Read the model definition and answer for the solid it produces. Units are mm, in the model's axes. A direction names the side the tool comes from. Round coordinates to 2 decimals unless told otherwise and drop trailing zeros.
from build123d import *

# Parameters (mm, degrees)
SKETCH2_W            = 37
SKETCH2_H            = 37
BOSS_EXTRUDE1_DEPTH  = 3
SKETCH3_R            = 6
BOSS_EXTRUDE2_DEPTH  = 2.3
SKETCH6_R            = 18.5
SKETCH6_R_2          = 8.5
BOSS_EXTRUDE3_DEPTH  = 2.3
CUT_EXTRUDE2_DEPTH   = 2.3
CIRPATTERN1_COUNT    = 4
CUT_EXTRUDE3_DEPTH   = 2.3
CIRPATTERN2_COUNT    = 4
CUT_EXTRUDE5_DEPTH   = 3
CIRPATTERN7_COUNT    = 4
MIRROR2_COPY_1_DEPTH = 3
MIRROR2_COPY_2_DEPTH = 3
MIRROR2_COPY_3_DEPTH = 3
SKETCH11_R           = 6.25
BOSS_EXTRUDE4_DEPTH  = 3
CIRPATTERN9_COUNT    = 2
CIRPATTERN9_ANGLE    = 90
SKETCH12_R           = 5
BOSS_EXTRUDE5_DEPTH  = 2.3
CIRPATTERN10_COUNT   = 2
CIRPATTERN10_ANGLE   = 90
CIRPATTERN11_COUNT   = 2
CIRPATTERN11_ANGLE   = 90
SCALE1_SCALE         = 0.965
SKETCH19_W           = 7
SKETCH19_H           = 6.5
CUT_EXTRUDE6_DEPTH   = 3
SKETCH20_W           = 5.6
SKETCH20_H           = 1.8
CUT_EXTRUDE7_DEPTH   = 1.5
SKETCH28_W           = 7
SKETCH28_H           = 6.5
CUT_EXTRUDE10_DEPTH  = 3
SKETCH30_W           = 5.6
SKETCH30_H           = 1.8
CUT_EXTRUDE11_DEPTH  = 1.5
CIRPATTERN12_COUNT   = 4
SKETCH33_W           = 7
SKETCH33_H           = 6.5
CUT_EXTRUDE12_DEPTH  = 3
SKETCH35_W           = 5.6
SKETCH35_H           = 1.8
CUT_EXTRUDE13_DEPTH  = 1.5
SKETCH37_W           = 7
SKETCH37_H           = 6.5
CUT_EXTRUDE14_DEPTH  = 3
SKETCH39_W           = 5.6
SKETCH39_H           = 1.8
CUT_EXTRUDE15_DEPTH  = 1.5


with BuildPart() as part:
    # Sketch2 → Boss-Extrude1 (new body)
    with BuildSketch(Plane.XY):
        Rectangle(SKETCH2_W, SKETCH2_H)
    extrude(amount=BOSS_EXTRUDE1_DEPTH)

    # Sketch3 → Boss-Extrude2 (add)
    with BuildSketch(Plane.XY.offset(3)):
        Circle(SKETCH3_R)
    extrude(amount=BOSS_EXTRUDE2_DEPTH)

    # Sketch5 → Revolve1 (revolve)
    with BuildSketch(Plane(origin=(0, 0, 0), x_dir=(-1, 0, 0), z_dir=(0, -1, 0))):
        with BuildLine():
            Line((6, -5.3), (0, -5.3))
            Line((0, -5.3), (0, -6.3))
            ThreePointArc((0, -6.3), (3.041381265, -6.048287591), (6, -5.3))
        make_face()
    revolve(axis=Axis((0, 0, 5.3), (0, 0, 1)))

    # Sketch6 → Boss-Extrude3 (add)
    with BuildSketch(Plane.XY.offset(3)):
        Circle(SKETCH6_R)
        Circle(SKETCH6_R_2, mode=Mode.SUBTRACT)
    extrude(amount=BOSS_EXTRUDE3_DEPTH)

    # Sketch8 → Cut-Extrude2 (cut)
    with BuildSketch(Plane.XY.offset(5.3)):
        with BuildLine():
            ThreePointArc((4.25, 7.361215932), (6.01040764, 6.01040764), (7.361215932, 4.25))
            Line((7.361215932, 4.25), (16.02146997, 9.25))
            ThreePointArc((16.02146997, 9.25), (13.081475452, 13.081475452), (9.25, 16.02146997))
            Line((9.25, 16.02146997), (4.25, 7.361215932))
        make_face()
    cut_extrude2 = extrude(amount=-CUT_EXTRUDE2_DEPTH, mode=Mode.SUBTRACT)

    # CirPattern1: Cut-Extrude2 ×4 about axis
    cirpattern1_axis = Axis((0, 0, 5.3), (0, 0, 1))
    for i in range(1, CIRPATTERN1_COUNT):
        add(cut_extrude2.rotate(cirpattern1_axis, i * 360 / CIRPATTERN1_COUNT), mode=Mode.SUBTRACT)

    # Sketch9 → Cut-Extrude3 (cut)
    with BuildSketch(Plane.XY.offset(5.3)):
        with BuildLine():
            Line((16.02146997, 9.25), (12.557368355, 7.25))
            Line((12.557368355, 7.25), (18.043966792, 4.082310915))
            ThreePointArc((18.043966792, 4.082310915), (17.227586832, 6.742421815), (16.02146997, 9.25))
        make_face()
        with BuildLine():
            Line((18.043966792, -4.082310915), (12.557368355, -7.25))
            Line((12.557368355, -7.25), (16.02146997, -9.25))
            ThreePointArc((16.02146997, -9.25), (17.227586832, -6.742421815), (18.043966792, -4.082310915))
        make_face()
    cut_extrude3 = extrude(amount=-CUT_EXTRUDE3_DEPTH, mode=Mode.SUBTRACT)

    # CirPattern2: Cut-Extrude3 ×4 about axis
    cirpattern2_axis = Axis((0, 0, 0), (0, 0, 1))
    for i in range(1, CIRPATTERN2_COUNT):
        add(cut_extrude3.rotate(cirpattern2_axis, i * 360 / CIRPATTERN2_COUNT), mode=Mode.SUBTRACT)

    # Sketch10 → Cut-Extrude5 (cut)
    with BuildSketch(Plane.XY.offset(3)):
        with BuildLine():
            Line((7.447468172, -12.671376657), (4.082310915, -18.5))
            Line((4.082310915, -18.5), (18.5, -18.5))
            Line((18.5, -18.5), (13.378483438, -13.378483438))
            ThreePointArc((13.378483438, -13.378483438), (12.288693225, -13.595256189), (11.671376657, -12.671376657))
            Line((11.671376657, -12.671376657), (7.447468172, -12.671376657))
        make_face()
    cut_extrude5 = extrude(amount=-CUT_EXTRUDE5_DEPTH, mode=Mode.SUBTRACT)

    # CirPattern7: Cut-Extrude5 ×4 about axis
    cirpattern7_axis = Axis((0, 0, 0), (0, 0, 1))
    for i in range(1, CIRPATTERN7_COUNT):
        add(cut_extrude5.rotate(cirpattern7_axis, i * 360 / CIRPATTERN7_COUNT), mode=Mode.SUBTRACT)

    # Mirror2: Cut-Extrude5 across plane
    add(cut_extrude5.mirror(Plane(origin=(0, 0, 0), x_dir=(0, 0, 1), z_dir=(0.707106781, -0.707106781, 0))), mode=Mode.SUBTRACT)

    # Mirror2 copy 1 sketch → Mirror2 copy 1 (cut)
    with BuildSketch(Plane.XY.offset(3)):
        with BuildLine():
            Line((7.447468172, 12.671376657), (4.082310915, 18.5))
            Line((4.082310915, 18.5), (18.5, 18.5))
            Line((18.5, 18.5), (13.378483438, 13.378483438))
            ThreePointArc((13.378483438, 13.378483438), (12.288693225, 13.595256189), (11.671376657, 12.671376657))
            Line((11.671376657, 12.671376657), (7.447468172, 12.671376657))
        make_face()
    extrude(amount=-MIRROR2_COPY_1_DEPTH, mode=Mode.SUBTRACT)

    # Mirror2 copy 2 sketch → Mirror2 copy 2 (cut)
    with BuildSketch(Plane(origin=(0, 0, 3), x_dir=(0, -1, 0), z_dir=(0, 0, 1))):
        with BuildLine():
            Line((7.447468172, 12.671376657), (4.082310915, 18.5))
            Line((4.082310915, 18.5), (18.5, 18.5))
            Line((18.5, 18.5), (13.378483438, 13.378483438))
            ThreePointArc((13.378483438, 13.378483438), (12.288693225, 13.595256189), (11.671376657, 12.671376657))
            Line((11.671376657, 12.671376657), (7.447468172, 12.671376657))
        make_face()
    extrude(amount=-MIRROR2_COPY_2_DEPTH, mode=Mode.SUBTRACT)

    # Mirror2 copy 3 sketch → Mirror2 copy 3 (cut)
    with BuildSketch(Plane(origin=(0, 0, 3), x_dir=(-1, 0, 0), z_dir=(0, 0, 1))):
        with BuildLine():
            Line((7.447468172, 12.671376657), (4.082310915, 18.5))
            Line((4.082310915, 18.5), (18.5, 18.5))
            Line((18.5, 18.5), (13.378483438, 13.378483438))
            ThreePointArc((13.378483438, 13.378483438), (12.288693225, 13.595256189), (11.671376657, 12.671376657))
            Line((11.671376657, 12.671376657), (7.447468172, 12.671376657))
        make_face()
    extrude(amount=-MIRROR2_COPY_3_DEPTH, mode=Mode.SUBTRACT)

    # Sketch11 → Boss-Extrude4 (add)
    with BuildSketch(Plane.XY):
        with Locations((14.849242405, 14.849242405)):
            Circle(SKETCH11_R)
    boss_extrude4 = extrude(amount=BOSS_EXTRUDE4_DEPTH)

    # CirPattern9: Boss-Extrude4 ×2 about axis
    cirpattern9_axis = Axis((0, 0, 5.3), (0, 0, 1))
    for i in range(1, CIRPATTERN9_COUNT):
        add(boss_extrude4.rotate(cirpattern9_axis, i * CIRPATTERN9_ANGLE / (CIRPATTERN9_COUNT - 1)))

    # Sketch12 → Boss-Extrude5 (add)
    with BuildSketch(Plane.XY.offset(3)):
        with Locations((14.849242405, 14.849242405)):
            Circle(SKETCH12_R)
    boss_extrude5 = extrude(amount=BOSS_EXTRUDE5_DEPTH)

    # Sketch14 → Revolve2 (revolve)
    with BuildSketch(Plane(origin=(14.849242405, 0, 0), x_dir=(0, 0, -1), z_dir=(1, 0, 0))):
        with BuildLine():
            Line((-6.3, 14.849242405), (-5.3, 14.849242405))
            Line((-5.3, 14.849242405), (-5.3, 9.849242405))
            ThreePointArc((-5.3, 9.849242405), (-6.047548784, 12.299732648), (-6.3, 14.849242405))
        make_face()
    revolve2 = revolve(axis=Axis((14.849242405, 14.849242405, 5.3), (0, 0, 1)))

    # CirPattern10: Boss-Extrude5 ×2 about axis
    cirpattern10_axis = Axis((0, 0, 5.3), (0, 0, 1))
    for i in range(1, CIRPATTERN10_COUNT):
        add(boss_extrude5.rotate(cirpattern10_axis, i * CIRPATTERN10_ANGLE / (CIRPATTERN10_COUNT - 1)))

    # CirPattern11: Revolve2 ×2 about axis
    cirpattern11_axis = Axis((0, 0, 5.3), (0, 0, 1))
    for i in range(1, CIRPATTERN11_COUNT):
        add(revolve2.rotate(cirpattern11_axis, i * CIRPATTERN11_ANGLE / (CIRPATTERN11_COUNT - 1)))


with BuildPart() as part_1:
    # Scale1: scaled about (0, 0, 0)
    add(part.part.scale(SCALE1_SCALE))

    # Sketch19 → Cut-Extrude6 (cut)
    with BuildSketch(Plane(origin=(0, 0, 0), x_dir=(-1, 0, 0), z_dir=(0, 0, -1))):
        Rectangle(SKETCH19_W, SKETCH19_H)
    extrude(amount=-CUT_EXTRUDE6_DEPTH, mode=Mode.SUBTRACT)

    # Sketch20 → Cut-Extrude7 (cut)
    with BuildSketch(Plane(origin=(0, 0, 0), x_dir=(-1, 0, 0), z_dir=(0, 0, -1))):
        with Locations((0, 4.15)):
            Rectangle(SKETCH20_W, SKETCH20_H)
        with Locations((0, -4.15)):
            Rectangle(SKETCH20_W, SKETCH20_H)
    extrude(amount=-CUT_EXTRUDE7_DEPTH, mode=Mode.SUBTRACT)

    # Sketch28 → Cut-Extrude10 (cut)
    with BuildSketch(Plane(origin=(-9.998493026, 1.351076982, 0), x_dir=(-1, 0, 0), z_dir=(0, 0, -1))):
        with Locations((1.751506974, -1.351076982)):
            Rectangle(SKETCH28_W, SKETCH28_H)
    cut_extrude10 = extrude(amount=-CUT_EXTRUDE10_DEPTH, mode=Mode.SUBTRACT)

    # Sketch30 → Cut-Extrude11 (cut)
    with BuildSketch(Plane(origin=(-9.998493026, 1.351076982, 0), x_dir=(-1, 0, 0), z_dir=(0, 0, -1))):
        with Locations((1.751506974, 2.798923018)):
            Rectangle(SKETCH30_W, SKETCH30_H)
        with Locations((1.751506974, -5.501076982)):
            Rectangle(SKETCH30_W, SKETCH30_H)
    cut_extrude11 = extrude(amount=-CUT_EXTRUDE11_DEPTH, mode=Mode.SUBTRACT)

    # CirPattern12: Cut-Extrude10, Cut-Extrude11 ×4 about axis
    cirpattern12_axis = Axis((0, 0, 0), (0, 0, 1))
    for i in range(1, CIRPATTERN12_COUNT):
        add(cut_extrude10.rotate(cirpattern12_axis, i * 360 / CIRPATTERN12_COUNT), mode=Mode.SUBTRACT)
        add(cut_extrude11.rotate(cirpattern12_axis, i * 360 / CIRPATTERN12_COUNT), mode=Mode.SUBTRACT)

    # Sketch33 → Cut-Extrude12 (cut)
    with BuildSketch(Plane(origin=(-14.368957264, 14.283753363, 0), x_dir=(-1, 0, 0), z_dir=(0, 0, -1))):
        with Locations((-0.039438343, 0.045765558)):
            Rectangle(SKETCH33_W, SKETCH33_H)
    extrude(amount=-CUT_EXTRUDE12_DEPTH, mode=Mode.SUBTRACT)

    # Sketch35 → Cut-Extrude13 (cut)
    with BuildSketch(Plane(origin=(-14.368957264, 14.283753363, 0), x_dir=(-1, 0, 0), z_dir=(0, 0, -1))):
        with Locations((-0.039438343, 4.195765558)):
            Rectangle(SKETCH35_W, SKETCH35_H)
        with Locations((-0.039438343, -4.104234442)):
            Rectangle(SKETCH35_W, SKETCH35_H)
    extrude(amount=-CUT_EXTRUDE13_DEPTH, mode=Mode.SUBTRACT)

    # Sketch37 → Cut-Extrude14 (cut)
    with BuildSketch(Plane(origin=(13.371321797, 14.128872217, 0), x_dir=(-1, 0, 0), z_dir=(0, 0, -1))):
        with Locations((-0.958197123, 0.200646703)):
            Rectangle(SKETCH37_W, SKETCH37_H)
    extrude(amount=-CUT_EXTRUDE14_DEPTH, mode=Mode.SUBTRACT)

    # Sketch39 → Cut-Extrude15 (cut)
    with BuildSketch(Plane(origin=(13.371321797, 14.128872217, 0), x_dir=(-1, 0, 0), z_dir=(0, 0, -1))):
        with Locations((-0.958197123, 4.350646703)):
            Rectangle(SKETCH39_W, SKETCH39_H)
        with Locations((-0.958197123, -3.949353297)):
            Rectangle(SKETCH39_W, SKETCH39_H)
    extrude(amount=-CUT_EXTRUDE15_DEPTH, mode=Mode.SUBTRACT)


solid = part_1.part
Q1. For a pull along X with two mould halves and no side action, classify faces 5 (the face through (14.73, 5.49, 4.02)), 6 (the face through (0, -12, 5.114)), 7 (the face through (-5.05, -12, 1)) as released by +X, released by -X, zero draft, split by the parting line, or undercut.
Outcome:
face 5: released by +X
face 6: zero draft
face 7: undercut
Q2. Flat-ended cylindrical pins translate along their axes: pin 1 (0.7 mm diameter, centred on x = 7.5, z = 2, fed in from +Y); pin 2 (3.5 mm diameter, centred on y = -10.5, z = 1, fed in from +X); pin 3 (1.6 mm diameter, centred on y = 10.5, z = 0.5, fed in from -X); pin 4 (1.5 mm diameter, centred on x = 16, y = 4.5, fed in from -Z). Find the tip coordinate at first contact, or state that the pin passes through.
Outcome:
pin 1: stops at y = 12.29
pin 2: stops at x = 13.19
pin 3: stops at x = -19.54
pin 4: stops at z = 0
Q3. Straight lines are drawn through the part: probe 1 along X at (y, z) = (-3, 2.25); probe 2 along X at (y, z) = (-11, 0.5); probe 3 along Y at (x, z) = (17.5, 0.75). For each, find the intervals that lie inside material, in ascending order.
Outcome:
probe 1: x = -17.85 to -15.25, -8.25 to -3.5, 3.5 to 8.25, 15.25 to 17.85
probe 2: x = -12.23 to -5.05, 5.05 to 12.23
probe 3: y = -4.14 to 4.14, 9.2 to 11.08, 17.58 to 19.46
Q4. For faces 1 (the face through (0, -5.05, 1)), 2 (the face through (2.9, 5.4, 2.895)), 3 (the face through (12.228, -9, 1)), 4 (the face through (5.586, 15.001, 1.468)), determine the directions among +Z, -Z, +X, -X, +Y, -Y from which every point of the face is accessible in a straight line to the end or side of a thin tool.
Outcome:
face 1: -Z
face 2: +Z
face 3: +Z, -Z, +X
face 4: +Z, -Z, +Y
